Design review of the part built by this model. Coordinates are the model's own, in mm. Give positions to 0.01 mm unless a question says otherwise; leave off trailing zeros. Loops run counter-clockwise (first coordinate to the right, second up) from the corner with the lowest first, then second, coordinate; pieces in that order, holes last. Notation, with made-up numbers: (-24, 81) -> (7, 81) arc R32 cw to (7, 107) -> close; hole circle Ø11 at (12.25, 77). An arc over 180 degrees is marked (long way). Answer in a Markdown table with one row per item. Add a question column.
(1) For line 1 (Z direction, x = -34, y = 5.5); line 2 (X direction, y = 3.75, z = -40.15); line 3 (X direction, y = 9.5, z = 30.5), list the stretches that pass through material, from the lowest coordinate up.
(2) Consider section B-B on x = -20. Write out the cut boundary in (y, z).
(3) Draft analysis for pull direction Y (two halves, no side actions). For faces 1 (the cylindrical face through (-0.547, 14.164, 0.646)), 2 (the cylindrical face through (31.32, 6.9, -1.04)), 3 (the conical face through (-0.77, 17.97, 31.08)), state which applies: +Y half, -Y half, draft (parallel to the pull), parting line (faces both ways), or undercut.
(4) Consider section A-A on y = 10. Write out the cut boundary in (x, z).
(5) Consider section C-C on x = -34. Count the separate pieces of the cut face and the enclosed holes in it, then the cut area to 3 significant figures.
(6) For pin 1 (7.5 mm diameter, centred on x = -34, z = -40.15, fed in from +Y), flat-tipped, find the tip position at first contact; note if it passes through.
(7) Consider section D-D on z = 20. Write out the cut boundary in (x, y).
from build123d import *
from OCP.BRepFilletAPI import BRepFilletAPI_MakeChamfer

# Parameters (mm, degrees)
SKETCH1_W                 = 80
SKETCH1_H                 = 92.3
BOSS_EXTRUDE1_DEPTH       = 20
HOLE1_D                   = 5.8
HOLE1_CBORE_D             = 6.5
HOLE1_CBORE_DEPTH         = 6
CHAMFER1_SIZE             = 6
CHAMFER1_SIZE_2           = 0.35
SKETCH4_R                 = 4.2
SKETCH4_R_2               = 5.1
CUT_EXTRUDE1_DEPTH        = 103.563590031
HOLE2_D                   = 4.8
HOLE2_CBORE_D             = 5.4
HOLE2_CBORE_DEPTH         = 4
CHAMFER2_SIZE2            = 0.3
CHAMFER2_SIZE             = 4
CHAMFER2_OF_MIRROR1_SIZE2 = 0.3
CHAMFER2_OF_MIRROR1_SIZE  = 4
FILLET1_R                 = 2


with BuildPart() as part:
    # Sketch1 → Boss-Extrude1 (new body)
    with BuildSketch(Plane(origin=(0, 0, 0), x_dir=(1, 0, 0), z_dir=(0, 1, 0))):
        Rectangle(SKETCH1_W, SKETCH1_H)
    extrude(amount=BOSS_EXTRUDE1_DEPTH)

    # Hole1 (through all)
    with Locations(Plane(origin=(0, 20, 0), x_dir=(1, 0, 0), z_dir=(0, 1, 0))):
        with Locations((-34, 40.15), (34, 40.15), (34, 2.15), (-34, 2.15)):
            CounterBoreHole(HOLE1_D / 2, HOLE1_CBORE_D / 2, HOLE1_CBORE_DEPTH)

    # Chamfer1
    chamfer1_edges_1 = [part.edges().sort_by_distance(p)[0] for p in [
        (-37.25, 14, -2.15),
    ]]
    chamfer1_side_1 = [part.faces().sort_by_distance(p)[0] for p in [
        (-37.25, 14.007, -2.15),
    ]]
    chamfer1_edges_2 = [part.edges().sort_by_distance(p)[0] for p in [
        (30.75, 14, -2.15),
    ]]
    chamfer1_side_2 = [part.faces().sort_by_distance(p)[0] for p in [
        (30.75, 14.007, -2.15),
    ]]
    chamfer1_edges_3 = [part.edges().sort_by_distance(p)[0] for p in [
        (30.75, 14, -40.15),
    ]]
    chamfer1_side_3 = [part.faces().sort_by_distance(p)[0] for p in [
        (30.75, 14.007, -40.15),
    ]]
    chamfer1_edges_4 = [part.edges().sort_by_distance(p)[0] for p in [
        (-37.25, 14, -40.15),
    ]]
    chamfer1_side_4 = [part.faces().sort_by_distance(p)[0] for p in [
        (-37.25, 14.007, -40.15),
    ]]
    chamfer1 = BRepFilletAPI_MakeChamfer(part.part.solid().wrapped)
    for e in chamfer1_edges_1:
        chamfer1.Add(CHAMFER1_SIZE - 0.0001, CHAMFER1_SIZE_2 - 0.0001, e.wrapped, chamfer1_side_1[0].wrapped)
    for e in chamfer1_edges_2:
        chamfer1.Add(CHAMFER1_SIZE - 0.0001, CHAMFER1_SIZE_2 - 0.0001, e.wrapped, chamfer1_side_2[0].wrapped)
    for e in chamfer1_edges_3:
        chamfer1.Add(CHAMFER1_SIZE - 0.0001, CHAMFER1_SIZE_2 - 0.0001, e.wrapped, chamfer1_side_3[0].wrapped)
    for e in chamfer1_edges_4:
        chamfer1.Add(CHAMFER1_SIZE - 0.0001, CHAMFER1_SIZE_2 - 0.0001, e.wrapped, chamfer1_side_4[0].wrapped)
    add(Compound.cast(chamfer1.Shape()), mode=Mode.REPLACE)  # a hair under: the kernel refuses the full size

    # Sketch4 → Cut-Extrude1 (cut, through all)
    with BuildSketch(Plane.XY.offset(46.15)):
        with Locations((0, 10)):
            Circle(SKETCH4_R)
        with Locations((-20, 10)):
            Circle(SKETCH4_R_2)
        with Locations((20, 10)):
            Circle(SKETCH4_R_2)
    extrude(amount=-CUT_EXTRUDE1_DEPTH, mode=Mode.SUBTRACT)

    # Hole2 (through all)
    with Locations(Plane(origin=(-40, 0, 0), x_dir=(0, 0, 1), z_dir=(0, -1, 0))):
        with Locations((28.65, -40)):
            hole2 = CounterBoreHole(HOLE2_D / 2, HOLE2_CBORE_D / 2, HOLE2_CBORE_DEPTH)

    # Chamfer2
    chamfer2_edges = [part.edges().sort_by_distance(p)[0] for p in [
        (0, 4, 25.95),
    ]]
    chamfer2_side = [part.faces().sort_by_distance(p)[0] for p in [
        (0, 3.994, 25.95),
    ]]
    chamfer(chamfer2_edges, length=CHAMFER2_SIZE - 0.0001, length2=CHAMFER2_SIZE2 - 0.0001, reference=chamfer2_side[0])  # a hair under: the kernel refuses the full size

    # Mirror1: Hole2 across plane
    add(hole2.mirror(Plane.ZX.offset(10)), mode=Mode.SUBTRACT)

    # Chamfer2 of Mirror1
    chamfer2_of_mirror1_edges = [part.edges().sort_by_distance(p)[0] for p in [
        (0, 16, 25.95),
    ]]
    chamfer2_of_mirror1_side = [part.faces().sort_by_distance(p)[0] for p in [
        (0, 16.006, 25.95),
    ]]
    chamfer(chamfer2_of_mirror1_edges, length=CHAMFER2_OF_MIRROR1_SIZE - 0.0001, length2=CHAMFER2_OF_MIRROR1_SIZE2 - 0.0001, reference=chamfer2_of_mirror1_side[0])  # a hair under: the kernel refuses the full size

    # Fillet1
    fillet1_edges = [part.edges().sort_by_distance(p)[0] for p in [
        (0, 0, 46.15),
        (-40, 0, 0),
        (0, 0, -46.15),
        (40, 0, 0),
        (40, 10, 46.15),
        (-40, 10, 46.15),
        (-40, 10, -46.15),
        (40, 10, -46.15),
    ]]
    fillet(fillet1_edges, radius=FILLET1_R)


solid = part.part
Values follow:
| question | item | result |
|---|---|---|
| 1 | line 1 | -46.15 to -43.05, -37.25 to -5.05, 0.75 to 46.15 |
| 1 | line 2 | -40 to -36.9, -31.1 to 31.1, 36.9 to 40 |
| 1 | line 3 | -40 to -25.08, -14.92 to -4.17, 4.17 to 14.92, 25.08 to 40 |
| 2 | outline | (0, -44.15) arc R2 ccw to (2, -46.15) -> (4.9, -46.15) -> (4.9, 46.15) -> (2, 46.15) arc R2 ccw to (0, 44.15) -> close; (15.1, -46.15) -> (20, -46.15) -> (20, 46.15) -> (15.1, 46.15) -> close |
| 3 | face 1 | undercut |
| 3 | face 2 | draft |
| 3 | face 3 | +Y half |
| 4 | outline | (-40, -44.15) arc R2 ccw to (-38, -46.15) -> (-25.1, -46.15) -> (-25.1, 46.15) -> (-38, 46.15) arc R2 ccw to (-40, 44.15) -> close; (-14.9, -46.15) -> (-4.2, -46.15) -> (-4.2, 46.15) -> (-14.9, 46.15) -> close; (4.2, -46.15) -> (14.9, -46.15) -> (14.9, 46.15) -> (4.2, 46.15) -> close; (25.1, -46.15) -> (38, -46.15) arc R2 ccw to (40, -44.15) -> (40, 44.15) arc R2 ccw to (38, 46.15) -> (25.1, 46.15) -> close; hole circle Ø5.8 at (-34, -40.15); hole circle Ø5.8 at (-34, -2.15); hole circle Ø5.8 at (34, -40.15); hole circle Ø5.8 at (34, -2.15) |
| 5 | separate pieces | 3 |
| 5 | enclosed holes | 0 |
| 5 | area | 1,610 mm2 |
| 6 | pin 1 | y = 20 |
| 7 | outline | (-40, 2) arc R2 ccw to (-38, 0) -> (38, 0) arc R2 ccw to (40, 2) -> (40, 20) -> (-40, 20) -> close; hole circle Ø10.2 at (-20, 10); hole circle Ø8.4 at (0, 10); hole circle Ø10.2 at (20, 10) |
